from build123d import *

# Parameters (mm, degrees)
SKETCH020_W          = 36.5
SKETCH020_H          = 19
PAD015_DEPTH         = 50
THICKNESS003_T       = 1
SKETCH021_W          = 11.43
SKETCH021_H          = 6.35
POCKET003_DEPTH      = 51.001
SKETCH022_W          = 6.35
SKETCH022_H          = 11.43
POCKET004_DEPTH      = 19.251
POCKET004_DEPTH_BACK = 19.251
SKETCH028_W          = 10
SKETCH028_H          = 25.4
SKETCH028_W_2        = 5
POCKET005_DEPTH      = 5
FILLET006_R          = 0.99
SKETCH034_W          = 36.5
SKETCH034_H          = 3.365
PAD021_DEPTH         = 4
CHAMFER_SIZE         = 1
CHAMFER001_SIZE      = 0.49


with BuildPart() as part:
    # Sketch020 → Pad015 (new body, symmetric)
    with BuildSketch(Plane.XY):
        Rectangle(SKETCH020_W, SKETCH020_H)
    extrude(amount=PAD015_DEPTH, both=True)

    # Thickness003
    thickness003_openings = [part.faces().sort_by_distance(p)[0] for p in [
        (0, 0, 50),
    ]]
    offset(amount=THICKNESS003_T, openings=thickness003_openings)

    # Sketch021 → Pocket003 (cut, through all)
    with BuildSketch(Plane.XY):
        with Locations((7.62, -2.96)):
            Rectangle(SKETCH021_W, SKETCH021_H)
        with Locations((-7.62, -2.96)):
            Rectangle(SKETCH021_W, SKETCH021_H)
    extrude(amount=-POCKET003_DEPTH, mode=Mode.SUBTRACT)

    # Sketch022 → Pocket004 (cut, two sides)
    with BuildSketch(Plane.YZ) as pocket004_sk:
        with Locations((-6.325, 43.285)):
            Rectangle(SKETCH022_W, SKETCH022_H)
    extrude(amount=-POCKET004_DEPTH, mode=Mode.SUBTRACT)
    extrude(pocket004_sk.sketch, amount=POCKET004_DEPTH_BACK, mode=Mode.SUBTRACT)

    # Sketch028 → Pocket005 (cut)
    with BuildSketch(Plane.XZ.offset(7)):
        with Locations((-23, 0)):
            Rectangle(SKETCH028_W, SKETCH028_H)
        with Locations((23, 0)):
            Rectangle(SKETCH028_W, SKETCH028_H)
        with Locations((-6.833333, 0)):
            Rectangle(SKETCH028_W_2, SKETCH028_H)
        with Locations((6.833333, 0)):
            Rectangle(SKETCH028_W_2, SKETCH028_H)
    extrude(amount=POCKET005_DEPTH, mode=Mode.SUBTRACT)

    # Fillet006
    fillet006_edges = [part.edges().sort_by_distance(p)[0] for p in [
        (-18, -9.5, 0),
        (-9.333333, -9.5, 0),
        (-4.333333, -10.5, 0),
        (4.333333, -10.5, 0),
        (9.333333, -9.5, 0),
        (18, -9.5, 0),
    ]]
    fillet(fillet006_edges, radius=FILLET006_R)

    # Sketch034 → Pad021 (join)
    with BuildSketch(Plane.XY.offset(-50)):
        with Locations((0, -7.8175)):
            Rectangle(SKETCH034_W, SKETCH034_H)
        with Locations((0, 1.8975)):
            Rectangle(SKETCH034_W, SKETCH034_H)
    extrude(amount=PAD021_DEPTH)

    # Chamfer
    chamfer_edges = [part.edges().sort_by_distance(p)[0] for p in [
        (0, 0.215, -46),
        (0, -6.135, -46),
    ]]
    chamfer(chamfer_edges, length=CHAMFER_SIZE)

    # Chamfer001
    chamfer001_edges = [part.edges().sort_by_distance(p)[0] for p in [
        (0, -9.5, 50),
        (-18.25, 0, 50),
        (0, 9.5, 50),
        (18.25, 0, 50),
    ]]
    chamfer(chamfer001_edges, length=CHAMFER001_SIZE)


solid = part.part
Here's how the part is built. I have some questions about the finished solid (model axes, mm). A direction names the side the tool comes from. Coordinates: 2 decimals unless noted, no trailing zeros. Order: outer loops, then holes, each group sorted by start corner. A loop starts at its lowest first (then second) coordinate and runs counter-clockwise, first axis right, second up. Notation, with made-up numbers: (29.5, 50.25) - (70.5, 50.25) arc R3 ccw to (70.5, 54.25) - close; hole circle Ø11 at (-33, 85.25). An arc over 180 degrees is marked (long way). Use CSV: the item, a comma, the result in double quotes. Start each with the question number.
1. Suppose I cut it at B-B on z = 42. List the corners of the cut face in (x, y) for me.
2. For faces 1 (the face through (0, 2, -46)), 2 (the face through (-0.1, 10.2, 50)), which set-ups out of +Z, -Z, +X, -X, +Y, -Y let a thin tool reach every point of the face, with its end or its side?
3. I'm going to push flat-ended pins straight in: pin 1 (1.9 mm diameter, centred on x = 0, y = -4.5, fed in from +Z); pin 2 (0.8 mm diameter, centred on y = -2.5, z = -50.5, fed in from +X) (3 decimals). Where does each tip first touch, or does it pass through?
4. Suppose I cut it at D-D on z = -1. Give the number of separate pieces and of enclosed holes in the cut face, then the cut area to 3 significant figures.
5. Suppose I cut it at C-C on y = -2.25. List the corners of the cut face in (x, z) for me (3 decimals), then the cut area to 3 significant figures.
6. Please list where these lines run through material, in increasing order: line 1 (X direction, y = 8.5, z = -32); line 2 (Y direction, x = -16.5, z = -3); line 3 (Z direction, x = -2.5, y = 9.25). Write a range as from..to.
7. Suppose I cut it at A-A on x = -12. List the corners of the cut face in (y, z) for me (3 decimals), then the cut area to 3 significant figures.
8. If we mould it in two halves opening along Y, with no side actions, what happens to faces 3 (the face through (-19.25, 0, 1)), 4 (the face through (16, -3, -50)), 5 (the face through (0, 10.5, 1)), 6 (the face through (0, -3, -50))? For each: +Y half, -Y half, draft (parallel to the pull), parting line (faces both ways), or undercut.
Output:
1,outline,"(-19.25, -9.5) arc R1 ccw to (-18.25, -10.5) - (18.25, -10.5) arc R1 ccw to (19.25, -9.5) - close; (-19.25, -3.15) - (-18.25, -3.15) - (-18.25, 9.5) - (18.25, 9.5) - (18.25, -3.15) - (19.25, -3.15) - (19.25, 9.5) arc R1 ccw to (18.25, 10.5) - (-18.25, 10.5) arc R1 ccw to (-19.25, 9.5) - close"
2,face 1,"+Z"
2,face 2,"+Z, +X, -X, +Y, -Y"
3,pin 1,"stops at z = -50"
3,pin 2,"stops at x = 19.245"
4,separate pieces,"4"
4,enclosed holes,"0"
4,area,"95.8 mm2"
5,outline,"(-19.25, -50) arc R1 ccw to (-18.25, -51) - (-13.335, -51) - (-13.335, -50) - (-18.25, -50) - (-18.25, 49.51) - (-18.74, 50) - (-19.25, 50) - close; (-1.905, -51) - (1.905, -51) - (1.905, -50) - (-1.905, -50) - close; (13.335, -51) - (18.25, -51) arc R1 ccw to (19.25, -50) - (19.25, 50) - (18.74, 50) - (18.25, 49.51) - (18.25, -50) - (13.335, -50) - close"
5,area,"215 mm2"
6,line 1,"x = -19.25..-18.25, 18.25..19.25"
6,line 2,"y = -10.5..-9.5, 9.5..10.5"
6,line 3,"z = -51..-50"
7,outline,"(-10.5, -50) arc R1 ccw to (-9.5, -51) - (-6.135, -51) - (-6.135, -47) - (-7.135, -46) - (-9.5, -46) - (-9.5, 49.51) - (-9.99, 50) - (-10.5, 50) - close; (0.215, -51) - (9.5, -51) arc R1 ccw to (10.5, -50) - (10.5, 50) - (9.99, 50) - (9.5, 49.51) - (9.5, -50) - (3.58, -50) - (3.58, -46) - (1.215, -46) - (0.215, -47) - close"
7,area,"240 mm2"
8,face 3,"draft"
8,face 4,"undercut"
8,face 5,"+Y half"
8,face 6,"undercut"
